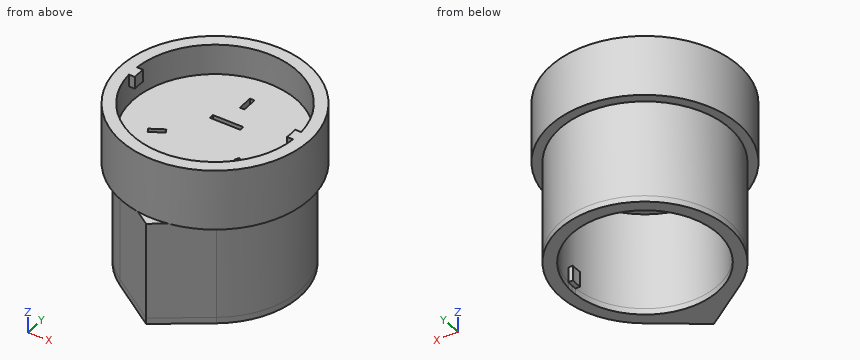
from build123d import *

# Parameters (mm, degrees)
F0_R      = 14
F0_R_2    = 12
F1_DEPTH  = 16
F3_DEPTH  = 2.5
F4_R      = 15.5
F5_DEPTH  = 5
F6_W      = 5
F6_H      = 0.75
F6_W_2    = 0.375
F6_H_2    = 2.5
F7_DEPTH  = 5.001
F8_R      = 15.5
F8_R_2    = 13.5
F9_DEPTH  = 5
F11_DEPTH = 2
F13_DEPTH = 16
F15_DEPTH = 1


with BuildPart() as f1:
    # F0 (on Top) → F1 (new body)
    with BuildSketch(Plane.XY):
        Circle(F0_R)
        Circle(F0_R_2, mode=Mode.SUBTRACT)
    extrude(amount=F1_DEPTH)

    # F2 (on Top) → F3 (join)
    with BuildSketch(Plane.XY):
        with BuildLine():
            Line((-11.2159206042, 0.875), (-11.968056442, 0.875))
            ThreePointArc((-11.968056442, 0.875), (-12, 0), (-11.968056442, -0.875))
            Line((-11.968056442, -0.875), (-11.2159206042, -0.875))
            ThreePointArc((-11.2159206042, -0.875), (-11.25, 0), (-11.2159206042, 0.875))
        make_face()
        with BuildLine():
            ThreePointArc((11.968056442, -0.875), (12, 0), (11.968056442, 0.875))
            Line((11.968056442, 0.875), (11.2159206042, 0.875))
            ThreePointArc((11.2159206042, 0.875), (11.25, 0), (11.2159206042, -0.875))
            Line((11.2159206042, -0.875), (11.968056442, -0.875))
        make_face()
    extrude(amount=F3_DEPTH)

    # F4 (on face) → F5 (join)
    with BuildSketch(Plane.XY.offset(16)):
        Circle(F4_R)
    extrude(amount=F5_DEPTH)

    # F6 (on face) → F7 (cut, through all)
    with BuildSketch(Plane(origin=(0, 0, 16), x_dir=(1, 0, 0), z_dir=(0, 0, -1))):
        with Locations((0, -2.8625)):
            Rectangle(F6_W, F6_H)
        with Locations((0.1875, -7.9375)):
            Rectangle(F6_W_2, F6_H_2)
        with Locations((-0.1875, -7.9375)):
            Rectangle(F6_W_2, F6_H_2)
        Polygon((5.6040448878, 3.6685095264), (5.7915448878, 3.34375), (7.9566083973, 4.59375), (7.7691083973, 4.9185095264), align=None)
        Polygon((7.9566083973, 4.59375), (5.7915448878, 3.34375), (5.9790448878, 3.0189904736), (8.1441083973, 4.2689904736), align=None)
        Polygon((-5.9790448878, 3.0189904736), (-5.7915448878, 3.34375), (-7.9566083973, 4.59375), (-8.1441083973, 4.2689904736), align=None)
        Polygon((-7.9566083973, 4.59375), (-5.7915448878, 3.34375), (-5.6040448878, 3.6685095264), (-7.7691083973, 4.9185095264), align=None)
    extrude(amount=-F7_DEPTH, mode=Mode.SUBTRACT)

    # F8 (on face) → F9 (join)
    with BuildSketch(Plane.XY.offset(21)):
        Circle(F8_R)
        Circle(F8_R_2, mode=Mode.SUBTRACT)
    extrude(amount=F9_DEPTH)

    # F10 (on face) → F11 (join)
    with BuildSketch(Plane.XY.offset(26)):
        with BuildLine():
            Line((-12.4599357944, 1), (-13.4629120178, 1))
            ThreePointArc((-13.4629120178, 1), (-13.5, 0), (-13.4629120178, -1))
            Line((-13.4629120178, -1), (-12.4599357944, -1))
            ThreePointArc((-12.4599357944, -1), (-12.5, 0), (-12.4599357944, 1))
        make_face()
        with BuildLine():
            Line((13.4629120178, 1), (12.4599357944, 1))
            ThreePointArc((12.4599357944, 1), (12.5, 0), (12.4599357944, -1))
            Line((12.4599357944, -1), (13.4629120178, -1))
            ThreePointArc((13.4629120178, -1), (13.5, 0), (13.4629120178, 1))
        make_face()
    extrude(amount=-F11_DEPTH)

    # F12 (on face) → F13 (join, through all)
    with BuildSketch(Plane(origin=(0, 0, 16), x_dir=(1, 0, 0), z_dir=(0, 0, -1))):
        with BuildLine():
            ThreePointArc((-7.9418300385, 11.5294117647), (0, 14), (7.9418300385, 11.5294117647))
            Line((7.9418300385, 11.5294117647), (0, 17))
            Line((0, 17), (-7.9418300385, 11.5294117647))
        make_face()
    extrude(amount=F13_DEPTH)

    # F14 (on face) → F15 (join)
    with BuildSketch(Plane(origin=(0, 0, 0), x_dir=(1, 0, 0), z_dir=(0, 0, -1))):
        with BuildLine():
            ThreePointArc((-7.9418300385, 11.5294117647), (0, -14), (7.9418300385, 11.5294117647))
            Line((7.9418300385, 11.5294117647), (0, 17))
            Line((0, 17), (-7.9418300385, 11.5294117647))
        make_face()
        with BuildLine():
            ThreePointArc((11.968056442, 0.875), (11.9920114515, 0.4377914432), (12, 0))
            ThreePointArc((12, 0), (11.9920114515, -0.4377914432), (11.968056442, -0.875))
            ThreePointArc((11.968056442, -0.875), (0, -12), (-11.968056442, -0.875))
            ThreePointArc((-11.968056442, -0.875), (-12, 0), (-11.968056442, 0.875))
            ThreePointArc((-11.968056442, 0.875), (0, 12), (11.968056442, 0.875))
        make_face(mode=Mode.SUBTRACT)
    extrude(amount=F15_DEPTH)


solid = f1.part
Work out the finished part from the listing and answer in its coordinate system (mm). Coordinates: 2 decimals unless noted, no trailing zeros. Loops run counter-clockwise (first coordinate to the right, second up) from the corner with the lowest first, then second, coordinate; pieces in that order, holes last. Notation, with made-up numbers: M 2,53 L 37,53 A24 cw 37,84 Z; hole C 1.25,43 d2. An arc over 180 degrees is marked long. Answer in a Markdown table with one row per item. Add a question column.
1. Find section B-B, the plane x = 13. Write down the section's boundary in (y, z).
2. Find section C-C, the plane z = 17.75. Write down the section's boundary in (x, y) (1 decimal).
3. Find section D-D, the plane y = 5. Write down the section's boundary in (x, z).
4. Flat-ended cylindrical pins translate along their axes: P1, Ø5.5, axis at x = -1, z = 18, coming from the +Y side; P2, Ø1.5, axis at y = 10, z = 14.5, coming from the +X side; P3, Ø12, axis at x = 1, y = 4.5, coming from the -Z side; P4, Ø13.5, axis at x = 1.5, y = -1, coming from the +Z side. Find the tip coordinate at first contact, or state that the pin passes through.
5. Consider L1, parallel to Y at x = 0, z = 24.35; L2, parallel to X at y = 0, z = 12.5. Determine where each line is inside the solid, lowest interval first.
6. Find section A-A, the plane z = 1.5. Write down the section's boundary in (x, y) (3 decimals).
Reported:
| question | item | result |
|---|---|---|
| 1 | outline | M -8.44,16 L -5.2,16 L -5.2,-1 L 5.2,-1 L 5.2,16 L 8.44,16 L 8.44,26 L 3.64,26 L 3.64,21 L -3.64,21 L -3.64,26 L -8.44,26 Z; M -1,24 L 1,24 L 1,26 L -1,26 Z |
| 2 | outline | C 0,0 d31; hole M -8.1,-4.3 L -7.8,-4.9 L -5.6,-3.7 L -6,-3 Z; hole M -2.5,2.5 L 2.5,2.5 L 2.5,3.2 L -2.5,3.2 Z; hole M -0.4,6.7 L 0.4,6.7 L 0.4,9.2 L -0.4,9.2 Z; hole M 5.6,-3.7 L 7.8,-4.9 L 8.1,-4.3 L 6,-3 Z |
| 3 | outline | M -14.67,16 L -13.08,16 L -13.08,-1 L -10.91,-1 L -10.91,16 L 10.91,16 L 10.91,-1 L 13.08,-1 L 13.08,16 L 14.67,16 L 14.67,26 L 12.54,26 L 12.54,21 L -12.54,21 L -12.54,26 L -14.67,26 Z |
| 4 | P1 | stops at y = 15.5 |
| 4 | P2 | stops at x = 10.51 |
| 4 | P3 | stops at z = 16 |
| 4 | P4 | stops at z = 21 |
| 5 | L1 | y = -15.5 to -13.5, 13.5 to 15.5 |
| 5 | L2 | x = -14 to -12, 12 to 14 |
| 6 | outline | M -7.942,-11.529 L 0,-17 L 7.942,-11.529 A14 ccw long Z; hole M -11.968,-0.875 A12 ccw 11.968,-0.875 L 11.216,-0.875 A11.25 ccw 11.216,0.875 L 11.968,0.875 A12 ccw -11.968,0.875 L -11.216,0.875 A11.25 ccw -11.216,-0.875 Z |
